Can you work these out from the drawing? Everything is in mm from the part's minimum corner. A direction names the side the tool comes from. Give positions to 0.01 mm unless a question says otherwise; leave off trailing zeros. Loops run counter-clockwise (first coordinate to the right, second up) from the corner with the lowest first, then second, coordinate; pieces in that order, holes last.
Q1. If we section it at C-C (y = 2.5): Please give me the cut outline in (x, z), plus the area to 3 significant figures.
Q2. Will this pin go through, and if not, where does the flat tip stop? P1, Ø1, axis at x = 44.5, z = 60.5, coming from the -Y side.
Q3. For the marked faces 1 and 2, which set-ups out of +Z, -Z, +X, -X, +Y, -Y let a thin tool reach every point of the face, with its end or its side?
Q4. If we section it at A-A (z = 34): Please give me the cut outline in (x, y).
Q5. We'd pull the mould along X, two halves only. Please class the marked faces 3, 4, 5 and 6: +X half, -X half, draft (parallel to the pull), parting line (faces both ways), or undercut.
Q6. If we section it at B-B (x = 6.5): Please give me the cut outline in (y, z).
Q7. I need wall thicknesses on line 1 (Z direction, x = 73.5, y = 10.5); line 2 (Y direction, x = 33, z = 92). Which ranges of each line are inside material? Lowest first, please.
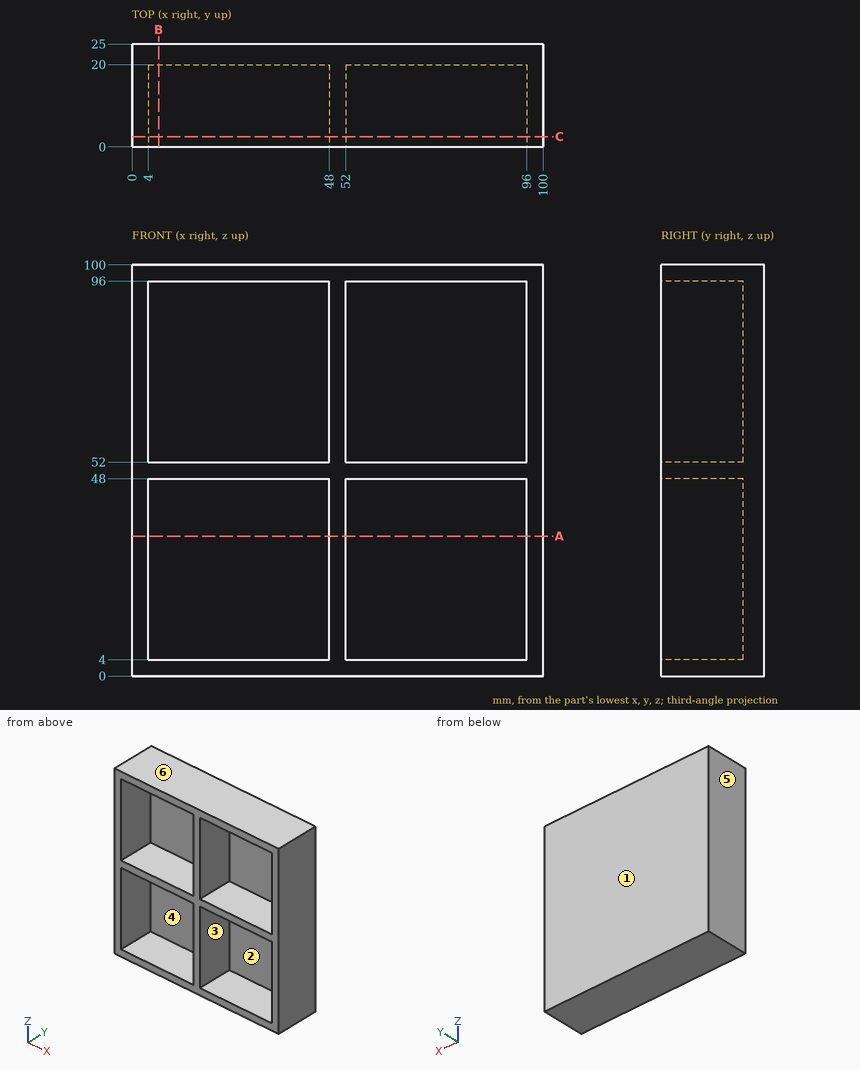
Check sheet entries:
1. outline: (0, 0) - (100, 0) - (100, 100) - (0, 100) - close; hole (4, 4) - (48, 4) - (48, 48) - (4, 48) - close; hole (4, 52) - (48, 52) - (48, 96) - (4, 96) - close; hole (52, 4) - (96, 4) - (96, 48) - (52, 48) - close; hole (52, 52) - (96, 52) - (96, 96) - (52, 96) - close
1. area: 2,260 mm2
2. P1: stops at y = 20
3. face 1: +Z, -Z, +X, -X, +Y
3. face 2: -Y
4. outline: (0, 0) - (4, 0) - (4, 20) - (48, 20) - (48, 0) - (52, 0) - (52, 20) - (96, 20) - (96, 0) - (100, 0) - (100, 25) - (0, 25) - close
5. face 3: undercut
5. face 4: undercut
5. face 5: -X half
5. face 6: draft
6. outline: (0, 0) - (25, 0) - (25, 100) - (0, 100) - (0, 96) - (20, 96) - (20, 52) - (0, 52) - (0, 48) - (20, 48) - (20, 4) - (0, 4) - close
7. line 1: z = 0 to 4, 48 to 52, 96 to 100
7. line 2: y = 20 to 25
